The model under review builds one solid part; all positions refer to its coordinate system, in mm. A direction names the side the tool comes from. Round coordinates to 2 decimals unless told otherwise and drop trailing zeros. Write each loop counter-clockwise with the first axis right and the second up, starting at its lowest first coordinate (ties: lowest second). Pieces come first, ordered by that corner, then holes. Notation, with made-up numbers: (15.25, -24) - (72.25, -24) arc R24 cw to (72.25, 3) - close; hole circle Ø4 at (-23, -6.75). An arc over 180 degrees is marked (long way). Write each question's results on one line, items separated by ' | '.
```python
from build123d import *

# Parameters (mm, degrees)
SKETCH020_W     = 6
SKETCH020_H     = 35
PAD004_DEPTH    = 31
SKETCH021_R     = 11.2
POCKET_DEPTH    = 6.001
FILLET004_R     = 1
SKETCH027_R     = 0.75
POCKET009_DEPTH = 12


with BuildPart() as part:
    # Sketch020 → Pad004 (new body)
    with BuildSketch(Plane.XY):
        with Locations((70, 5)):
            Rectangle(SKETCH020_W, SKETCH020_H)
    extrude(amount=PAD004_DEPTH)

    # Sketch021 → Pocket (cut, through all)
    with BuildSketch(Plane.YZ.offset(73)):
        with Locations((5, 31)):
            Circle(SKETCH021_R)
    extrude(amount=-POCKET_DEPTH, mode=Mode.SUBTRACT)

    # Fillet004
    fillet004_edges = [part.edges().sort_by_distance(p)[0] for p in [
        (73, -12.5, 15.5),
        (67, -12.5, 15.5),
        (70, -12.5, 0),
        (70, -12.5, 31),
        (67, 22.5, 15.5),
        (73, 22.5, 15.5),
        (70, 22.5, 0),
        (70, 22.5, 31),
    ]]
    fillet(fillet004_edges, radius=FILLET004_R)

    # Sketch027 → Pocket009 (cut)
    with BuildSketch(Plane.XY.offset(31)):
        with Locations((70, 18.85)):
            Circle(SKETCH027_R)
        with Locations((70, -8.85)):
            Circle(SKETCH027_R)
    extrude(amount=-POCKET009_DEPTH, mode=Mode.SUBTRACT)


solid = part.part
```
Q1. Tool access review of faces 4 (the cylindrical face through (67.285, 22.199, 15.717)), 5 (the cylindrical face through (69.25, 18.88, 25.08)): name each direction out of +Z, -Z, +X, -X, +Y, -Y from which nothing blocks a thin tool from reaching the whole face with its end or side.
Evaluation:
face 4: +Z, -Z, -X, +Y | face 5: +Z
Q2. We need section B-B (x = 70). State the section outline as (y, z) points.
Evaluation:
outline: (-12.5, 1) arc R1 ccw to (-11.5, 0) - (21.5, 0) arc R1 ccw to (22.5, 1) - (22.5, 30) arc R1 ccw to (21.5, 31) - (19.6, 31) - (19.6, 19) - (18.1, 19) - (18.1, 31) - (16.2, 31) arc R11.2 cw to (-6.2, 31) - (-8.1, 31) - (-8.1, 19) - (-9.6, 19) - (-9.6, 31) - (-11.5, 31) arc R1 ccw to (-12.5, 30) - close
Q3. For probe 1 along Y at (x, z) = (70, 24); probe 2 along Y at (x, z) = (68.9, 26.5); probe 3 along Y at (x, z) = (72.1, 19), list the stretches that pass through material, from the lowest coordinate up.
Evaluation:
probe 1: y = -12.5 to -9.6, -8.1 to -3.74, 13.74 to 18.1, 19.6 to 22.5 | probe 2: y = -12.5 to -5.26, 15.26 to 22.5 | probe 3: y = -12.49 to 22.49
Q4. The part is to be moulded in two halves that separate along Y. For faces 1 (the cylindrical face through (70.042, -12.199, 30.715)), 2 (the cylindrical face through (70.042, 22.215, 30.699)), 3 (the cylindrical face through (70, 4.8, 19.8)), say which applies: released by +Y, released by -Y, zero draft, split by the parting line, or undercut.
Evaluation:
face 1: released by -Y | face 2: released by +Y | face 3: undercut
Q5. We need section D-D (z = 25.5). State the section outline as (x, y) points, plus the area to 3 significant figures.
Evaluation:
outline: (67, -11.5) arc R1 ccw to (68, -12.5) - (72, -12.5) arc R1 ccw to (73, -11.5) - (73, -4.76) - (67, -4.76) - close; (67, 14.76) - (73, 14.76) - (73, 21.5) arc R1 ccw to (72, 22.5) - (68, 22.5) arc R1 ccw to (67, 21.5) - close; hole circle Ø1.5 at (70, -8.85); hole circle Ø1.5 at (70, 18.85) | area: 88.5 mm^2
Q6. We need section C-C (y = 18.85). State the section outline as (x, z) points.
Evaluation:
outline: (67, 0) - (73, 0) - (73, 31) - (70.75, 31) - (70.75, 19) - (69.25, 19) - (69.25, 31) - (67, 31) - close
Q7. We need section A-A (z = 29.5). State the section outline as (x, y) points.
Evaluation:
outline: (67, -11.5) arc R1 ccw to (68, -12.5) - (72, -12.5) arc R1 ccw to (73, -11.5) - (73, -6.1) - (67, -6.1) - close; (67, 16.1) - (73, 16.1) - (73, 21.5) arc R1 ccw to (72, 22.5) - (68, 22.5) arc R1 ccw to (67, 21.5) - close; hole circle Ø1.5 at (70, -8.85); hole circle Ø1.5 at (70, 18.85)
